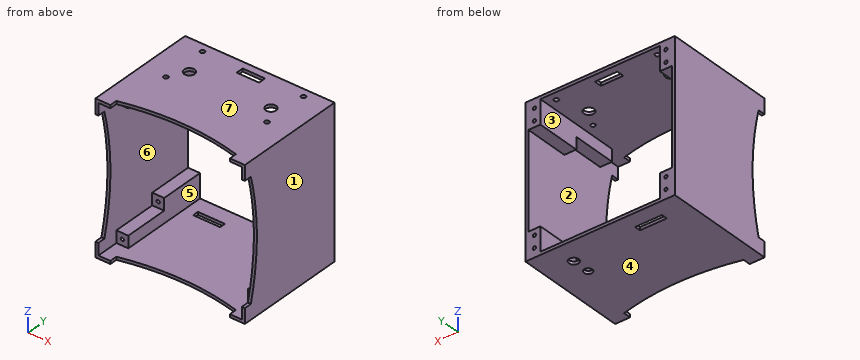
Autodesk Inventor part; units mm, degrees
ref_plane "YZ Plane" through (0, 0, 0) normal (1, 0, 0) x (0, 1, 0)
ref_plane "XZ Plane" through (0, 0, 0) normal (0, 1, 0) x (-1, 0, 0)
ref_plane "XY Plane" through (0, 0, 0) normal (0, 0, 1) x (1, 0, 0)
sketch "Skizze1" plane through (0, 0, 0) normal (0, 1, 0) x (-1, 0, 0)
  line L0 (-50, 50) -> (50, 50)
  line L1 (50, 50) -> (50, -50)
  line L2 (50, -50) -> (-50, -50)
  line L3 (-50, -50) -> (-50, 50)
  line L4 (-50, 50) -> (50, -50) construction
  line L5 (50, 50) -> (-50, -50) construction
  point P0 (0, 0)
  dimension "d0" = 100
  dimension "d1" = 100
extrude "Extrusion1" add sketch "Skizze1" along normal blind 75
sketch "Skizze2" plane through (0, 0, 0) normal (1, 0, 0) x (0, 1, 0)
  line L0 (5, 40) -> (0, 40)
  line L1 (0, 40) -> (0, -40)
  line L2 (0, -40) -> (5, -40)
  arc A0 (5, -40) -> (5, 40) centre (-152.5, 0) ccw
  point P0 (0, 0)
  point P1 (0, 0)
  dimension "d4" = 5
  dimension "d6" = 80
  dimension "d30" = 10
extrude "Extrusion2" cut sketch "Skizze2" along normal through all both and the other way through all
sketch "Skizze3" plane through (0, 0, 0) normal (0, 0, 1) x (1, 0, 0)
  line L0 (-40, 5) -> (-40, 0)
  line L1 (-40, 0) -> (40, 0)
  line L2 (40, 0) -> (40, 5)
  arc A0 (40, 5) -> (-40, 5) centre (0, -152.5) ccw
  point P0 (0, 0)
  point P1 (0, 0)
  point P2 (0, 0)
  dimension "d9" = 5
  dimension "d11" = 80
  dimension "d29" = 10
extrude "Extrusion3" cut sketch "Skizze3" along normal through all both and the other way through all
sketch "Skizze9" plane through (0, 75, 0) normal (0, 1, 0) x (1, 0, 0)
  line L0 (-50, -50) -> (50, -50)
  line L1 (50, -50) -> (50, 50)
  line L2 (50, 50) -> (-50, 50)
  line L3 (-50, 50) -> (-50, -50)
  line L4 (-48, -48) -> (48, -48)
  line L5 (48, -48) -> (48, 48)
  line L6 (48, 48) -> (-48, 48)
  line L7 (-48, 48) -> (-48, -48)
  line L8 (-40, 40) -> (-48, 40)
  line L9 (-48, 40) -> (-48, 48)
  line L10 (-48, 48) -> (-40, 48)
  line L11 (-40, 48) -> (-40, 40)
  line L12 (-40, 40) -> (-48, 48) construction
  line L13 (-48, 40) -> (-40, 48) construction
  line L14 (40, 40) -> (48, 40)
  line L15 (48, 40) -> (48, 48)
  line L16 (48, 48) -> (40, 48)
  line L17 (40, 48) -> (40, 40)
  line L18 (40, 40) -> (48, 48) construction
  line L19 (48, 40) -> (40, 48) construction
  line L20 (40, -40) -> (48, -40)
  line L21 (48, -40) -> (48, -48)
  line L22 (48, -48) -> (40, -48)
  line L23 (40, -48) -> (40, -40)
  line L24 (40, -40) -> (48, -48) construction
  line L25 (48, -40) -> (40, -48) construction
  line L26 (40, -32) -> (48, -32)
  line L27 (48, -32) -> (48, -40)
  line L28 (48, -40) -> (40, -40)
  line L29 (40, -40) -> (40, -32)
  line L30 (40, -32) -> (48, -40) construction
  line L31 (48, -32) -> (40, -40) construction
  line L32 (-40, 32) -> (-48, 32)
  line L33 (-48, 32) -> (-48, 40)
  line L34 (-48, 40) -> (-40, 40)
  line L35 (-40, 40) -> (-40, 32)
  line L36 (-40, 32) -> (-48, 40) construction
  line L37 (-48, 32) -> (-40, 40) construction
  line L38 (40, 32) -> (48, 32)
  line L39 (48, 32) -> (48, 40)
  line L40 (48, 40) -> (40, 40)
  line L41 (40, 40) -> (40, 32)
  line L42 (40, 32) -> (48, 40) construction
  line L43 (48, 32) -> (40, 40) construction
  line L44 (-40, -40) -> (-48, -40)
  line L45 (-48, -40) -> (-48, -48)
  line L46 (-48, -48) -> (-40, -48)
  line L47 (-40, -48) -> (-40, -40)
  line L48 (-40, -40) -> (-48, -48) construction
  line L49 (-48, -40) -> (-40, -48) construction
  line L50 (-40, -32) -> (-48, -32)
  line L51 (-48, -32) -> (-48, -40)
  line L52 (-48, -40) -> (-40, -40)
  line L53 (-40, -40) -> (-40, -32)
  line L54 (-40, -32) -> (-48, -40) construction
  line L55 (-48, -32) -> (-40, -40) construction
  point P0 (0, 0)
  point P1 (-44, 44)
  point P2 (44, 44)
  point P3 (44, -44)
  point P4 (44, -36)
  point P5 (-44, 36)
  point P6 (44, 36)
  point P7 (-44, -44)
  point P8 (-44, -36)
  point P9 (-44, 44)
  point P10 (-44, 36)
  point P11 (44, 44)
  point P12 (44, 36)
  point P13 (-44, -36)
  point P14 (-44, -44)
  point P15 (44, -36)
  point P16 (44, -44)
  dimension "d65" = 2
  dimension "d81" = 8
  dimension "d82" = 8
extrude "Extrusion9" cut sketch "Skizze9" against normal through all contours L7 L44 L47 L4 | L47 L53 L50 L7 L32 L35 L11 L6 L17 L41 L38 L5 L26 L29 L23 L4 | L7 L50 L53 L44 | L23 L20 L5 L4 | L29 L26 L5 L20 | L7 L8 L35 L32 | L7 L6 L11 L8 | L38 L41 L14 L5 | L14 L17 L6 L5
extrude "Extrusion10" add sketch "Skizze9" against normal blind 60 contours L7 L44 L47 L4 | L23 L20 L5 L4 | L7 L6 L11 L8 | L14 L17 L6 L5
extrude "Extrusion11" add sketch "Skizze9" against normal blind 30 contours L7 L50 L53 L44 | L29 L26 L5 L20 | L7 L8 L35 L32 | L38 L41 L14 L5
hole "Bohrung3" at (-44, 75, 44) at (-44, 75, 36) at (-44, 75, -36) at (-44, 75, -44) at (44, 75, -44) at (44, 75, -36) at (44, 75, 36) at (44, 75, 44) direction (0, -1, 0) diameter 2.2 end through all
sketch "Skizze10" plane through (0, -152.5, -48) normal (0, 0, 1) x (1, 0, 0)
  line L0 (-40, 227.5) -> (40, 227.5)
  circle A0 centre (30, 212) radius 3.25
  circle A1 centre (30, 200) radius 2.75
  line L1 (-33, 217) -> (-15, 217)
  line L2 (-15, 217) -> (-15, 213)
  line L3 (-15, 213) -> (-33, 213)
  line L4 (-33, 213) -> (-33, 217)
  line L5 (-33, 217) -> (-15, 213) construction
  line L6 (-15, 217) -> (-33, 213) construction
  line L7 (-48, 227.5) -> (-40, 227.5)
  line L8 (-48, 197.5) -> (-48, 227.5)
  line L9 (-40, 197.5) -> (-48, 197.5)
  line L10 (-40, 227.5) -> (-40, 197.5)
  line L11 (40, 227.5) -> (48, 227.5)
  line L12 (40, 227.5) -> (40, 197.5)
  line L13 (48, 197.5) -> (40, 197.5)
  line L14 (48, 227.5) -> (48, 197.5)
  point P0 (0, 152.5)
  point P1 (-24, 215)
  dimension "d83" = 6.5
  dimension "d84" = 15.5
  dimension "d85" = 18
  dimension "d86" = 5.5
  dimension "d87" = 2.5
  dimension "d89" = 15
  dimension "d90" = 18
  dimension "d91" = 4
  dimension "d92" = 15.5
extrude "Extrusion12" cut sketch "Skizze10" against normal up to surface (2 mm away) contours A0 | A1 | L1 L2 L3 L4
sketch "Skizze8" plane through (0, -142.5, 48) normal (0, 0, -1) x (-1, 0, 0)
  line L0 (-40, 217.5) -> (40, 217.5)
  line L1 (-7.5, 212.5) -> (7.5, 212.5)
  line L2 (7.5, 212.5) -> (7.5, 207.5)
  line L3 (7.5, 207.5) -> (-7.5, 207.5)
  line L4 (-7.5, 207.5) -> (-7.5, 212.5)
  circle A0 centre (27.3, 192.7) radius 3.4544
  circle A1 centre (-27.3, 192.7) radius 3.5
  circle A2 centre (27.3, 192.7) radius 3.5
  circle A3 centre (-27.3, 192.7) radius 3.4544
  circle A4 centre (-33.8, 211.8) radius 1.1
  circle A5 centre (-33.8, 181.2) radius 1.1
  circle A6 centre (33.8, 211.8) radius 1.1
  circle A7 centre (33.8, 181.2) radius 1.1
  circle A8 centre (-33.8, 211.8) radius 1.5
  circle A9 centre (33.8, 211.8) radius 1.5
  circle A10 centre (33.8, 181.2) radius 1.5
  circle A11 centre (-33.8, 181.2) radius 1.5
  point P0 (0, 152.5)
  point P1 (0, 212.5)
  point P2 (0, 217.5)
  point P3 (-40, 147.5)
  point P4 (40, 147.5)
  dimension "d57" = 15
  dimension "d58" = 5
  dimension "d59" = 5
  dimension "d60" = 7
  dimension "d61" = 7
  dimension "d64" = 3
extrude "Extrusion8" cut sketch "Skizze8" against normal up to surface (2 mm away) contours L1 L2 L3 L4 | A0 | A1 | A2 | A3 | A4 | A5 | A6 | A7 | A8 | A9 | A10 | A11
properties part number "DayLightGlow_Base"
Can you work these out from the model? Positions are in its coordinate system, mm. Face numbers are marked on the shaded views. A direction names the side the tool comes from. Round coordinates to 2 decimals unless told otherwise and drop trailing zeros. Write each loop counter-clockwise with the first axis right and the second up, starting at its lowest first coordinate (ties: lowest second). Pieces come first, ordered by that corner, then holes. Notation, with made-up numbers: (85, 19.25) - (96, 19.25) arc R18 ccw to (96, 34.25) - close; hole circle Ø6 at (45, -20.75). An arc over 180 degrees is marked (long way). Write each question's results on one line, items separated by ' | '. Start each with the question number.
1) Suppose I cut it at A-A (y = 17.5). List the corners of the cut face in (x, z) for me.
2) Which directions (+Z, -Z, +X, -X, +Y, -Y) give clear straight access to the entire face, cutting with the end or side of a thin tool? Please do the marked faces 5, 6 and 7.
3) Suppose I cut it at B-B (z = -20). List the corners of the cut face in (x, y) for me.
4) For pin 1 Ø9 at (x, z) = (-43, -38) entering from -Y, with a flat end and sliding along its axis, tell me the tip position at first contact or that it passes through.
5) Suppose I cut it at D-D (x = -27). List the corners of the cut face in (y, z) for me, and give its area (3 significant figures).
6) We'd pull the mould along X, two halves only. Please class the marked faces 1, 2, 3 and 4: released by +X, released by -X, zero draft, split by the parting line, or undercut.
7) Suppose I cut it at C-C (x = -9). List the corners of the cut face in (y, z) for me.
8) Please list where these lines run through material, in increasing order: line 1 (Z direction, x = 44, y = 58.5); line 2 (X direction, y = 69.3, z = 49.2); line 3 (X direction, y = 65, z = 36).
Here are the results:
1) outline: (-50, -50) - (50, -50) - (50, 50) - (-50, 50) - close; hole (-48, -40) - (-40, -40) - (-40, -48) - (40, -48) - (40, -40) - (48, -40) - (48, 40) - (40, 40) - (40, 48) - (-40, 48) - (-40, 40) - (-48, 40) - close; hole circle Ø2.2 at (-44, -44); hole circle Ø2.2 at (-44, 44); hole circle Ø2.2 at (44, -44); hole circle Ø2.2 at (44, 44)
2) face 5: +Y, -Y | face 6: -Y | face 7: +Z, +X, -X, +Y, -Y
3) outline: (-50, 8.76) - (-48, 8.76) - (-48, 75) - (-50, 75) - close; (48, 8.76) - (50, 8.76) - (50, 75) - (48, 75) - close
4) pin 1: stops at y = 15
5) outline: (7.74, -50) - (60.5, -50) - (60.5, -48) - (7.74, -48) - close; (7.74, 48) - (46.71, 48) - (46.71, 50) - (7.74, 50) - close; (53.69, 48) - (75, 48) - (75, 50) - (53.69, 50) - close; (64.5, -50) - (75, -50) - (75, -48) - (64.5, -48) - close | area: 247 mm2
6) face 1: released by +X | face 2: undercut | face 3: undercut | face 4: zero draft
7) outline: (9.75, -50) - (75, -50) - (75, -48) - (9.75, -48) - close; (9.75, 48) - (75, 48) - (75, 50) - (9.75, 50) - close
8) line 1: z = -50 to -45.1, -42.9 to -37.1, -34.9 to -32, 32 to 34.9, 37.1 to 42.9, 45.1 to 50 | line 2: x = -50 to -35.3, -32.3 to -7.5, 7.5 to 32.3, 35.3 to 50 | line 3: x = -50 to -45.1, -42.9 to -40, 40 to 42.9, 45.1 to 50
